from build123d import *

# Parameters (mm, degrees)
SKETCH_R        = 2
PAD_DEPTH       = 2.6
SKETCH001_W     = 57.7
SKETCH001_H     = 3.9
POCKET_DEPTH    = 5
SKETCH002_W     = 115.6
SKETCH002_H     = 5.2
POCKET001_DEPTH = 0.2
SKETCH003_W     = 118
SKETCH003_H     = 7.6
SKETCH003_W_2   = 115.6
SKETCH003_H_2   = 5.2
PAD001_DEPTH    = 2
SKETCH004_R     = 2.25
SKETCH004_R_2   = 1.7
SKETCH004_R_3   = 3.1
POCKET002_DEPTH = 5
SKETCH005_W     = 42
SKETCH005_H     = 1.2
POCKET003_DEPTH = 2
SKETCH006_W     = 15
SKETCH006_H     = 15
POCKET004_DEPTH = 2


with BuildPart() as part:
    # Sketch → Pad (new body)
    with BuildSketch(Plane.XY):
        with BuildLine():
            ThreePointArc((-4.134472, 4.620188), (-6.2, 0), (-4.134472, -4.620188))
            Line((-4.134472, -4.620188), (7.8, -15.3))
            Line((7.8, -15.3), (125.8, -15.3))
            Line((125.8, -15.3), (137.734472, -4.620188))
            ThreePointArc((137.734472, -4.620188), (139.8, 0), (137.734472, 4.620188))
            Line((125.8, 15.3), (137.734472, 4.620188))
            Line((7.8, 15.3), (125.8, 15.3))
            Line((-4.134472, 4.620188), (7.8, 15.3))
        make_face()
        Circle(SKETCH_R, mode=Mode.SUBTRACT)
        with Locations((133.6, 0)):
            Circle(SKETCH_R, mode=Mode.SUBTRACT)
    extrude(amount=PAD_DEPTH)

    # Sketch001 (on Face12 of Pad) → Pocket (cut)
    with BuildSketch(Plane.XY.offset(2.6)):
        with Locations((53.15, -13.35)):
            Rectangle(SKETCH001_W, SKETCH001_H)
    extrude(amount=-POCKET_DEPTH, mode=Mode.SUBTRACT)

    # Sketch002 (on Face4 of Pocket) → Pocket001 (cut)
    with BuildSketch(Plane(origin=(0, 0, 0), x_dir=(1, 0, 0), z_dir=(0, 0, -1))):
        with Locations((66.8, -2.6)):
            Rectangle(SKETCH002_W, SKETCH002_H)
    extrude(amount=-POCKET001_DEPTH, mode=Mode.SUBTRACT)

    # Sketch003 (on Face4 of Pocket001) → Pad001 (join)
    with BuildSketch(Plane(origin=(0, 0, 0), x_dir=(1, 0, 0), z_dir=(0, 0, -1))):
        with Locations((66.8, -2.6)):
            Rectangle(SKETCH003_W, SKETCH003_H)
        with Locations((66.8, -2.6)):
            Rectangle(SKETCH003_W_2, SKETCH003_H_2, mode=Mode.SUBTRACT)
    extrude(amount=PAD001_DEPTH)

    # Sketch004 (on Face5 of Pad001) → Pocket002 (cut)
    with BuildSketch(Plane.XY.offset(2.6)):
        with Locations((24.3, -5)):
            Circle(SKETCH004_R)
        with Locations((31.8, -5)):
            Circle(SKETCH004_R)
        with Locations((17, -5)):
            Circle(SKETCH004_R_2)
        with Locations((72.1, -4.6)):
            Circle(SKETCH004_R_3)
        with BuildLine():
            Line((42.1, -1.2), (56.3, -1.2))
            ThreePointArc((56.5, -1.4), (56.441421, -1.258579), (56.3, -1.2))
            Line((56.5, -1.4), (56.5, -8.63))
            ThreePointArc((56.3, -8.83), (56.441421, -8.771421), (56.5, -8.63))
            Line((56.3, -8.83), (42.1, -8.83))
            ThreePointArc((41.9, -8.63), (41.958579, -8.771421), (42.1, -8.83))
            Line((41.9, -8.63), (41.9, -1.4))
            ThreePointArc((42.1, -1.2), (41.958579, -1.258579), (41.9, -1.4))
        make_face()
        with BuildLine():
            Line((92.6, -2.4), (115.4, -2.4))
            ThreePointArc((116.2, -3.2), (115.965685, -2.634315), (115.4, -2.4))
            Line((116.2, -3.2), (116.2, -8.6))
            ThreePointArc((115.4, -9.4), (115.965685, -9.165685), (116.2, -8.6))
            Line((115.4, -9.4), (92.6, -9.4))
            ThreePointArc((91.8, -8.6), (92.034315, -9.165685), (92.6, -9.4))
            Line((91.8, -8.6), (91.8, -3.2))
            ThreePointArc((92.6, -2.4), (92.034315, -2.634315), (91.8, -3.2))
        make_face()
    extrude(amount=-POCKET002_DEPTH, mode=Mode.SUBTRACT)

    # Sketch005 (on Face43 of Pocket002) → Pocket003 (cut)
    with BuildSketch(Plane(origin=(0, 0, -2), x_dir=(1, 0, 0), z_dir=(0, 0, -1))):
        with Locations((37.8, 0.6)):
            Rectangle(SKETCH005_W, SKETCH005_H)
    extrude(amount=-POCKET003_DEPTH, mode=Mode.SUBTRACT)

    # Sketch006 (on Face44 of Pocket003) → Pocket004 (cut)
    with BuildSketch(Plane(origin=(0, 0, -2), x_dir=(1, 0, 0), z_dir=(0, 0, -1))):
        with Locations((72.1, 4.6)):
            Rectangle(SKETCH006_W, SKETCH006_H)
    extrude(amount=-POCKET004_DEPTH, mode=Mode.SUBTRACT)


solid = part.part
The listing builds one solid part. Answer for the finished solid, in the listing's coordinates (mm). A direction names the side the tool comes from. Coordinates: 2 decimals unless noted, no trailing zeros. Write each loop counter-clockwise with the first axis right and the second up, starting at its lowest first coordinate (ties: lowest second). Pieces come first, ordered by that corner, then holes. Notation, with made-up numbers: (-9, 66.25) - (33, 66.25) arc R13 ccw to (33, 90.25) - close; hole circle Ø7 at (34.25, 25). An arc over 180 degrees is marked (long way). Put each result on its own line as item: value.
1. The part is cut by section B-B on z = 1.1. State how many separate pieces and enclosed holes the cut face has, plus the area to 3 significant figures.
Answer sheet:
separate pieces: 1
enclosed holes: 8
area: 3,510 mm^2
2. The part is cut by section D-D on y = 8. Give the vertices of the cut face in (x, z).
Answer sheet:
outline: (-0.36, 0) - (133.96, 0) - (133.96, 2.6) - (-0.36, 2.6) - close
3. The part is cut by section C-C on x = 72.1. Give the vertices of the cut face in (y, z), plus the area to 3 significant figures.
Answer sheet:
outline: (-11.4, 0) - (-7.7, 0) - (-7.7, 2.6) - (-11.4, 2.6) - close; (-1.5, 0) - (0, 0) - (0, 0.2) - (5.2, 0.2) - (5.2, -2) - (6.4, -2) - (6.4, 0) - (15.3, 0) - (15.3, 2.6) - (-1.5, 2.6) - close
area: 54.7 mm^2
4. A tool of negligible diameter and unlimited length cuts with its end or side. For faces 4 (the face through (116.2, -6, 1)), 5 (the face through (1.749, 9.885, 1.282)), 6 (the face through (24.3, -13, 1)), from which of +Z, -Z, +X, -X, +Y, -Y can it reach the whole face along a straight path? Write none if from no direction.
Answer sheet:
face 4: +Z, -Z
face 5: +Z, -Z, -X, +Y
face 6: +Z, -Z, -Y
5. Find the intervals of material crossed by line 1 along Y through (x, z) = (110.5, 0.9); line 2 along Y through (x, z) = (72, 0.35); line 3 along X through (y, z) = (-0.5, -0.35), in increasing order. Write a range as from..to.
Answer sheet:
line 1: y = -15.3..-9.4, -2.4..15.3
line 2: y = -11.4..-7.7, -1.5..15.3
line 3: x = 7.8..16.8, 58.8..64.6, 79.6..125.8
6. Determine the mould class of faces 1 (the face through (131.602, 0.088, 1.282)), 2 (the face through (139.8, -0.1, 1.3)), 3 (the face through (131.684, -10.035, 1.282)) for opening direction Y: pulls with the +Y half, pulls with the -Y half, needs draft (parallel to the pull), parting line crosses it, or undercut.
Answer sheet:
face 1: undercut
face 2: parting line crosses it
face 3: pulls with the -Y half
7. The part is cut by section A-A on x = 0. Give the vertices of the cut face in (y, z).
Answer sheet:
outline: (-8.32, 0) - (-2, 0) - (-2, 2.6) - (-8.32, 2.6) - close; (2, 0) - (8.32, 0) - (8.32, 2.6) - (2, 2.6) - close
8. Flat-ended cylindrical pins translate along their axes: pin 1 Ø5 at (x, y) = (14, 3.5) entering from -Z; pin 2 Ø2 at (y, z) = (-6.5, 1.5) entering from +X; pin 3 Ø2 at (y, z) = (-12.5, 1.5) entering from -X; pin 4 Ø1.8 at (y, z) = (2.5, -0.5) entering from -X. Find the tip coordinate at first contact, or state that the pin passes through.
Answer sheet:
pin 1: stops at z = -2
pin 2: stops at x = 136.75
pin 3: stops at x = 3.55
pin 4: stops at x = -5.95
